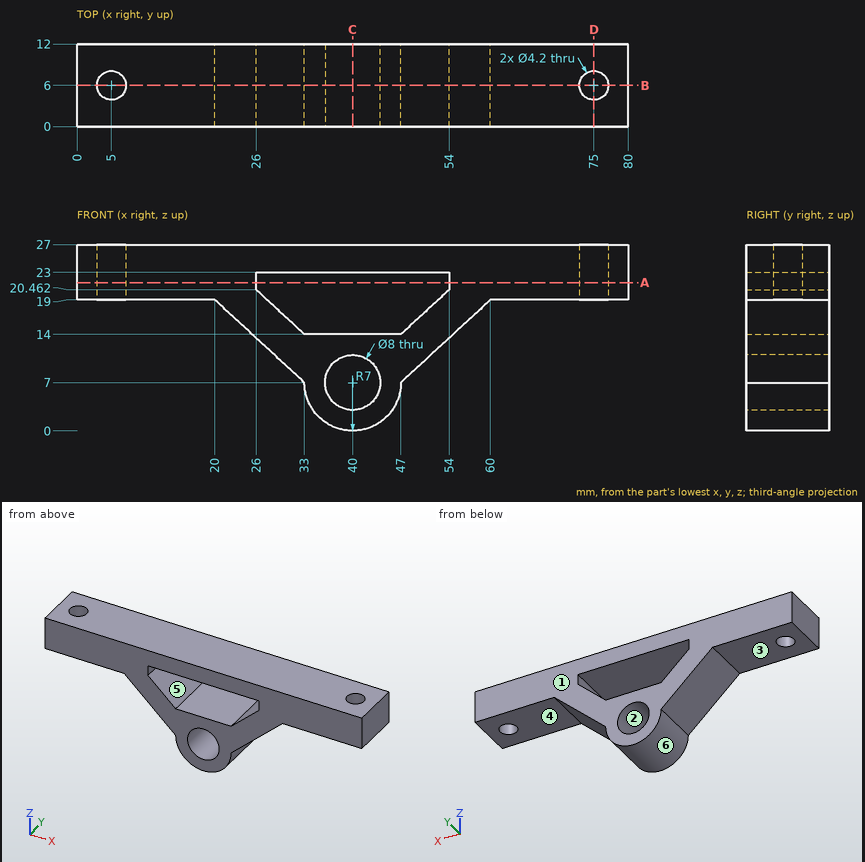
Part print with two shaded views. Sizes in mm from the minimum x, y, z corner. A direction names the side the tool comes from. Round coordinates to 2 decimals unless told otherwise and drop trailing zeros. Order: outer loops, then holes, each group sorted by start corner. A loop starts at its lowest first (then second) coordinate and runs counter-clockwise, first axis right, second up.
(1) Band-saw the part on C-C (x = 40). List the corners of the cut face in (y, z).
(2) 3-axis set-ups, long thin cutter, end or side, ignore diameter. For the marked faces 4, 5 and 6: which of +Z, -Z, +X, -X, +Y, -Y reach the whole face in a straight line?
(3) Band-saw the part on A-A (z = 21.5). List the corners of the cut face in (x, y).
(4) Band-saw the part on B-B (y = 6). List the corners of the cut face in (x, z).
(5) Pull direction Z, two halves, no side cores. Call the marked faces 1, 2 and 3: released by +Z, released by -Z, zero draft, split by the parting line, or undercut.
(6) Band-saw the part on D-D (x = 75). List the corners of the cut face in (y, z), then the cut area to 3 significant figures.
(7) Pin check, flat tips, straight feed: pin 1 (2 mm diameter, centred on y = 6, z = 14.5, fed in from +X); pin 2 (4 mm diameter, centred on y = 3, z = 3.5, fed in from -X); pin 3 (2.5 mm diameter, centred on x = 75, y = 6, fed in from +Z); pin 4 (3 mm diameter, centred on y = 7, z = 3, fed in from +X). Stop position of each tip, or through.
(8) Drill centre lines: line 1 (Z direction, x = 40, y = 4.5); line 2 (Y direction, x = 75, z = 23.25); line 3 (Z direction, x = 39, y = 0.75). Where is each one in solid material? Low to high.
Verdict:
1. outline: (0, 0) - (12, 0) - (12, 3) - (0, 3) - close; (0, 11) - (12, 11) - (12, 14) - (0, 14) - close; (0, 23) - (12, 23) - (12, 27) - (0, 27) - close
2. face 4: -Z, +X, +Y, -Y
2. face 5: +Y, -Y
2. face 6: -Z, +Y, -Y
3. outline: (0, 0) - (26, 0) - (26, 12) - (0, 12) - close; (54, 0) - (80, 0) - (80, 12) - (54, 12) - close; hole circle Ø4.2 at (5, 6); hole circle Ø4.2 at (75, 6)
4. outline: (0, 19) - (2.9, 19) - (2.9, 27) - (0, 27) - close; (7.1, 19) - (20, 19) - (33, 7) arc R7 ccw to (47, 7) - (60, 19) - (72.9, 19) - (72.9, 27) - (7.1, 27) - close; (77.1, 19) - (80, 19) - (80, 27) - (77.1, 27) - close; hole (26, 20.46) - (33, 14) - (47, 14) - (54, 20.46) - (54, 23) - (26, 23) - close; hole circle Ø8 at (40, 7)
5. face 1: zero draft
5. face 2: undercut
5. face 3: released by -Z
6. outline: (0, 19) - (3.9, 19) - (3.9, 27) - (0, 27) - close; (8.1, 19) - (12, 19) - (12, 27) - (8.1, 27) - close
6. area: 62.4 mm2
7. pin 1: stops at x = 56.21
7. pin 2: stops at x = 33.16
7. pin 3: passes through
7. pin 4: stops at x = 46.54
8. line 1: z = 0 to 3, 11 to 14, 23 to 27
8. line 2: y = 0 to 3.9, 8.1 to 12
8. line 3: z = 0.07 to 3.13, 10.87 to 14, 23 to 27
